```python
from build123d import *

# Parameters (mm, degrees)
F1_DEPTH = 25
F2_W     = 16
F2_H     = 20
F3_DEPTH = 26.601
F4_W     = 19.9722627059
F4_H     = 18.5
F5_DEPTH = 25.001
F6_R     = 1


with BuildPart() as f1:
    # F0 (on Top) → F1 (new body)
    with BuildSketch(Plane.XY):
        Polygon((-13.3, 40.5), (-13.3, 0), (0, 0), (13.3, 0), (13.3, 40.5), (10.3, 40.5), (10.3, 24.5), (0, 24.5), (-10.3, 24.5), (-10.3, 40.5), align=None)
    extrude(amount=F1_DEPTH)

    # F2 (on face) → F3 (cut, through all)
    with BuildSketch(Plane(origin=(-13.3, 0, 0), x_dir=(0, -1, 0), z_dir=(-1, 0, 0))):
        with Locations((-32.5, 15)):
            Rectangle(F2_W, F2_H)
    extrude(amount=-F3_DEPTH, mode=Mode.SUBTRACT)

    # F4 (on face) → F5 (cut, through all)
    with BuildSketch(Plane.XY):
        with Locations((-0.3138686471, 12.25)):
            Rectangle(F4_W, F4_H)
    extrude(amount=F5_DEPTH, mode=Mode.SUBTRACT)

    # F6
    f6_edges = [f1.edges().sort_by_distance(p)[0] for p in [
        (13.3, 20.25, 0),
        (13.3, 40.5, 2.5),
        (13.3, 32.5, 5),
        (13.3, 24.5, 15),
        (13.3, 12.25, 25),
        (13.3, 0, 12.5),
        (-13.3, 20.25, 0),
        (-13.3, 0, 12.5),
        (-13.3, 12.25, 25),
        (-13.3, 24.5, 15),
        (-13.3, 32.5, 5),
        (-13.3, 40.5, 2.5),
        (0, 0, 25),
        (0, 0, 0),
        (0, 24.5, 25),
        (0, 24.5, 0),
        (-11.8, 24.5, 5),
        (11.8, 24.5, 5),
        (10.3, 32.5, 5),
        (-10.3, 32.5, 0),
        (-10.3, 40.5, 2.5),
        (-10.3, 32.5, 5),
        (-10.3, 24.5, 2.5),
        (10.3, 32.5, 0),
        (10.3, 24.5, 2.5),
    ]]
    fillet(f6_edges, radius=F6_R)


solid = f1.part
```
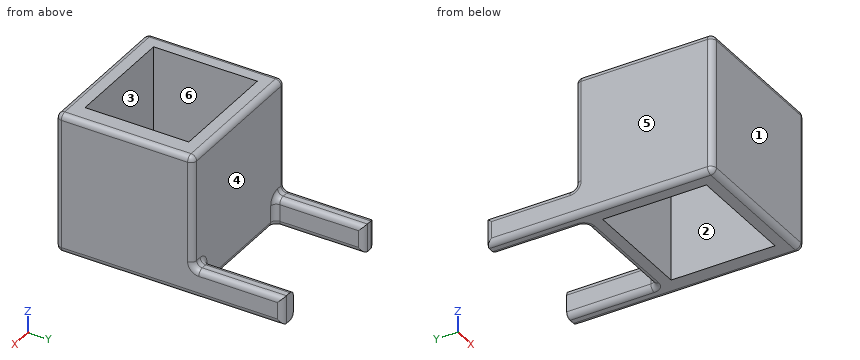
Design review of the part built by this model. Coordinates are the model's own, in mm. Face numbers are marked on the shaded views. A direction names the side the tool comes from. Give positions to 0.01 mm unless a question says otherwise; leave off trailing zeros. Order: outer loops, then holes, each group sorted by start corner. A loop starts at its lowest first (then second) coordinate and runs counter-clockwise, first axis right, second up. Notation, with made-up numbers: (80.25, -36) -> (126.25, -36) arc R8 ccw to (126.25, -23) -> close; hole circle Ø6 at (0.5, -16). An arc over 180 degrees is marked (long way). Write item = value, one per line. Start each with the question number.
(1) We need section A-A on x = 3.25. Write out the cut boundary in (y, z), plus the area to 3 significant figures.
(2) For pin 1 (7 mm diameter, centred on x = -2.5, z = 9.5, fed in from +Y); pin 2 (10 mm diameter, centred on y = 33.5, z = 17.5, fed in from -X); pin 3 (5 mm diameter, centred on x = -9.5, y = 18, fed in from -Z); pin 4 (6 mm diameter, centred on x = 9, y = 34, fed in from +Z), all flat-tipped, find the tip position at first contact; note any pin that passes through.
(3) For the marked faces 1 and 2, list the 3-axis set-ups (+Z, -Z, +X, -X, +Y, -Y) from which the entire face can be reached by the end or side of a thin tool; tool diameter is ignored.
(4) We need section C-C on z = 2.75. Write out the cut boundary in (x, y).
(5) We need section D-D on x = 11.75. Write out the cut boundary in (y, z), plus the area to 3 significant figures.
(6) To check wall thickness, follow line 1 along Y through (x, z) = (-3.75, 5.75); line 2 along X through (y, z) = (13.5, 2); line 3 along Y through (x, z) = (11.5, 22.25). State the ranges of each line that lie inside material, in increasing order.
(7) Mouldability with a two-part tool opening along Y and no side actions: class the marked faces 3, 4, 5 and 6 as +Y half, -Y half, draft (parallel to the pull), parting line (faces both ways), or undercut.
(8) We need section B-B on y = 8.5. Write out the cut boundary in (x, z), plus the area to 3 significant figures.
Numbers:
q1.outline = (0, 1) arc R1 ccw to (1, 0) -> (3, 0) -> (3, 25) -> (1, 25) arc R1 ccw to (0, 24) -> close; (21.5, 0) -> (23.5, 0) arc R1 ccw to (24.5, 1) -> (24.5, 24) arc R1 ccw to (23.5, 25) -> (21.5, 25) -> close
q1.area = 149 mm^2
q2.pin_1 = 24.5
q2.pin_2 = through
q2.pin_3 = 0
q2.pin_4 = 5
q3.face_1 = +Z, -Z, +X, -X, -Y
q3.face_2 = +Z, -Z
q4.outline = (-13.3, 1) arc R1 ccw to (-12.3, 0) -> (12.3, 0) arc R1 ccw to (13.3, 1) -> (13.3, 39.5) arc R1 ccw to (12.3, 40.5) -> (10.3, 40.5) -> (10.3, 25.5) arc R1 cw to (9.3, 24.5) -> (-9.3, 24.5) arc R1 cw to (-10.3, 25.5) -> (-10.3, 39.5) arc R1 ccw to (-11.3, 40.5) -> (-12.3, 40.5) arc R1 ccw to (-13.3, 39.5) -> close; hole (-10.3, 3) -> (9.67, 3) -> (9.67, 21.5) -> (-10.3, 21.5) -> close
q5.outline = (0, 1) arc R1 ccw to (1, 0) -> (40.5, 0) -> (40.5, 5) -> (25.5, 5) arc R1 cw to (24.5, 6) -> (24.5, 24) arc R1 ccw to (23.5, 25) -> (1, 25) arc R1 ccw to (0, 24) -> close
q5.area = 692 mm^2
q6.line_1 = 0 to 3, 21.5 to 24.5
q6.line_2 = -13.3 to -10.3, 9.67 to 13.3
q6.line_3 = 0 to 24.5
q7.face_3 = undercut
q7.face_4 = +Y half
q7.face_5 = draft
q7.face_6 = undercut
q8.outline = (-13.3, 1) arc R1 ccw to (-12.3, 0) -> (-10.3, 0) -> (-10.3, 25) -> (-12.3, 25) arc R1 ccw to (-13.3, 24) -> close; (9.67, 0) -> (12.3, 0) arc R1 ccw to (13.3, 1) -> (13.3, 24) arc R1 ccw to (12.3, 25) -> (9.67, 25) -> close
q8.area = 165 mm^2
